For this review, take the finished solid that the model builds, in its own axes (mm). Coordinates: 2 decimals unless noted, no trailing zeros. Loops run counter-clockwise (first coordinate to the right, second up) from the corner with the lowest first, then second, coordinate; pieces in that order, holes last. Notation, with made-up numbers: (-21.75, 82.5) - (-15.75, 82.5) arc R18 cw to (-15.75, 103.5) - close; hole circle Ø5 at (52, 35.5). An arc over 180 degrees is marked (long way). Use one line per item in the form item = value. Start each with the question number.
1. Add section D-D on x = 28.5. Give the boundary of the cut face in (y, z), and give its area (3 significant figures).
2. Draft analysis for pull direction X (two halves, no side actions). For faces 1 (the face through (-1, -20, -63.5)), 2 (the face through (6.481, -19, -38)), state which applies: +X half, -X half, draft (parallel to the pull), parting line (faces both ways), or undercut.
3. Add section C-C on x = -21. Give the boundary of the cut face in (y, z), and give its area (3 significant figures).
4. For pin 1 Ø12.5 at (x, z) = (-17.5, -2.5) entering from +Y, flat-tipped, find the tip position at first contact; note if it passes through.
5. Add section A-A on y = -36.5. Count the separate pieces of the cut face and the enclosed holes in it, and give its area (3 significant figures).
6. Add section B-B on z = -2.5. Give the boundary of the cut face in (x, y), and give its area (3 significant figures).
7. To check wall thickness, follow probe 1 along Z at (x, y) = (-14, -2.5); probe 2 along X at (y, z) = (-3.5, 3); probe 3 along X at (y, z) = (-25.5, 39). State the ranges of each line that lie inside material, in increasing order.
```python
from build123d import *

# Parameters (mm, degrees)
F0_W     = 76.46276
F0_H     = 127
F2_DEPTH = 40.64
F1_W     = 25.4
F1_H     = 25.4
F1_W_2   = 25.226503
F3_DEPTH = 38.1
F4_R     = 5.08


with BuildPart() as f2:
    # F0 (on Front) → F2 (new body)
    with BuildSketch(Plane.XZ):
        Rectangle(F0_W, F0_H)
    extrude(amount=F2_DEPTH)

    # F1 (on face) → F3 (cut)
    with BuildSketch(Plane.XZ):
        with Locations((-17.70053, 38.1)):
            Rectangle(F1_W, F1_H)
        with Locations((19.007883, 38.1)):
            Rectangle(F1_W, F1_H)
        with Locations((17.666091, 0)):
            Rectangle(F1_W, F1_H)
        with Locations((-17.890041, 0)):
            Rectangle(F1_W, F1_H)
        with Locations((-17.206696, -38.1)):
            Rectangle(F1_W, F1_H)
        with Locations((19.094631, -38.1)):
            Rectangle(F1_W_2, F1_H)
    extrude(amount=F3_DEPTH, mode=Mode.SUBTRACT)

    # F4
    f4_edges = [f2.edges().sort_by_distance(p)[0] for p in [
        (6.307883, -19.05, 25.4),
        (31.707883, -19.05, 25.4),
    ]]
    fillet(f4_edges, radius=F4_R)


solid = f2.part
```
Conclusion:
q1.outline = (-40.64, -63.5) - (0, -63.5) - (0, -50.8) - (-38.1, -50.8) - (-38.1, -25.4) - (0, -25.4) - (0, -12.7) - (-38.1, -12.7) - (-38.1, 12.7) - (0, 12.7) - (0, 25.76) - (-38.1, 25.76) - (-38.1, 50.8) - (0, 50.8) - (0, 63.5) - (-40.64, 63.5) - close
q1.area = 2,270 mm^2
q2.face_1 = draft
q2.face_2 = undercut
q3.outline = (-40.64, -63.5) - (0, -63.5) - (0, -50.8) - (-38.1, -50.8) - (-38.1, -25.4) - (0, -25.4) - (0, -12.7) - (-38.1, -12.7) - (-38.1, 12.7) - (0, 12.7) - (0, 25.4) - (-38.1, 25.4) - (-38.1, 50.8) - (0, 50.8) - (0, 63.5) - (-40.64, 63.5) - close
q3.area = 2,260 mm^2
q4.pin_1 = -38.1
q5.separate_pieces = 1
q5.enclosed_holes = 6
q5.area = 5,860 mm^2
q6.outline = (-38.23, -40.64) - (38.23, -40.64) - (38.23, 0) - (30.37, 0) - (30.37, -38.1) - (4.97, -38.1) - (4.97, 0) - (-5.19, 0) - (-5.19, -38.1) - (-30.59, -38.1) - (-30.59, 0) - (-38.23, 0) - close
q6.area = 1,170 mm^2
q7.probe_1 = -63.5 to -50.8, -25.4 to -12.7, 12.7 to 25.4, 50.8 to 63.5
q7.probe_2 = -38.23 to -30.59, -5.19 to 4.97, 30.37 to 38.23
q7.probe_3 = -38.23 to -30.4, -5 to 6.31, 31.71 to 38.23
